from build123d import *

# Parameters (mm, degrees)
F0_R     = 7.5
F1_DEPTH = 10
F2_DEPTH = 30


with BuildPart() as f1:
    # F0 (on Front) → F1 (new body)
    with BuildSketch(Plane.XZ):
        with BuildLine():
            ThreePointArc((3, -19.77372), (15.165751, -13.038405), (20, 0))
            ThreePointArc((20, 0), (15.165751, 13.038405), (3, 19.77372))
            ThreePointArc((3, 19.77372), (-20, 0), (3, -19.77372))
        make_face()
        with BuildLine():
            Line((12.5, 3), (12.5, -3))
            Line((12.5, -3), (6.873864, -3))
            ThreePointArc((6.873864, -3), (0, -7.5), (-6.873864, -3))
            Line((-6.873864, -3), (-12.5, -3))
            Line((-12.5, -3), (-12.5, 3))
            Line((-12.5, 3), (-6.873864, 3))
            ThreePointArc((-6.873864, 3), (0, 7.5), (6.873864, 3))
            Line((6.873864, 3), (12.5, 3))
        make_face(mode=Mode.SUBTRACT)
        with BuildLine():
            ThreePointArc((3, 19.77372), (15.165751, 13.038405), (20, 0))
            ThreePointArc((20, 0), (15.165751, -13.038405), (3, -19.77372))
            Line((3, -19.77372), (51.875, -12.358575))
            ThreePointArc((51.875, -12.358575), (37.5, 0), (51.875, 12.358575))
            Line((51.875, 12.358575), (3, 19.77372))
        make_face()
        with BuildLine():
            ThreePointArc((62.5, 0), (59.478594, 8.149003), (51.875, 12.358575))
            ThreePointArc((51.875, 12.358575), (37.5, 0), (51.875, -12.358575))
            ThreePointArc((51.875, -12.358575), (59.478594, -8.149003), (62.5, 0))
        make_face()
        with Locations((50, 0)):
            Circle(F0_R, mode=Mode.SUBTRACT)
        with BuildLine():
            Line((-12.5, -3), (-6.873864, -3))
            ThreePointArc((-6.873864, -3), (-7.5, 0), (-6.873864, 3))
            Line((-6.873864, 3), (-12.5, 3))
            Line((-12.5, 3), (-12.5, -3))
        make_face()
    extrude(amount=F1_DEPTH)

    # F0 (on Front) → F2 (join)
    with BuildSketch(Plane.XZ):
        with BuildLine():
            ThreePointArc((3, -19.77372), (15.165751, -13.038405), (20, 0))
            ThreePointArc((20, 0), (15.165751, 13.038405), (3, 19.77372))
            ThreePointArc((3, 19.77372), (-20, 0), (3, -19.77372))
        make_face()
        with BuildLine():
            Line((12.5, 3), (12.5, -3))
            Line((12.5, -3), (6.873864, -3))
            ThreePointArc((6.873864, -3), (0, -7.5), (-6.873864, -3))
            Line((-6.873864, -3), (-12.5, -3))
            Line((-12.5, -3), (-12.5, 3))
            Line((-12.5, 3), (-6.873864, 3))
            ThreePointArc((-6.873864, 3), (0, 7.5), (6.873864, 3))
            Line((6.873864, 3), (12.5, 3))
        make_face(mode=Mode.SUBTRACT)
        with BuildLine():
            Line((-12.5, -3), (-6.873864, -3))
            ThreePointArc((-6.873864, -3), (-7.5, 0), (-6.873864, 3))
            Line((-6.873864, 3), (-12.5, 3))
            Line((-12.5, 3), (-12.5, -3))
        make_face()
    extrude(amount=F2_DEPTH)


solid = f1.part
Can you work these out from the model? Positions are in its coordinate system, mm. A direction names the side the tool comes from. Round coordinates to 2 decimals unless told otherwise and drop trailing zeros. Order: outer loops, then holes, each group sorted by start corner. A loop starts at its lowest first (then second) coordinate and runs counter-clockwise, first axis right, second up. Notation, with made-up numbers: (-7, 22) -> (38, 22) arc R24 cw to (38, 48) -> close; hole circle Ø6 at (24, 19.5). An arc over 180 degrees is marked (long way). Write each question's results on one line, items separated by ' | '. Start each with the question number.
Item 1: Thinking about a two-plate mould opening in Z: for faces 3 (the flat face through (27.095, -4.93, -16.118)), 4 (the flat face through (12.5, -15, 0)), 5 (the flat face through (32, -10, 0)), 6 (the flat face through (27.78, -4.93, 16.014)), which applies, +Z half, -Z half, draft (parallel to the pull), parting line (faces both ways), or undercut?
Item 2: If we section it at C-C, the plane z = 5.5: Write out the boundary of the cut face in (x, y).
Item 3: Please list where these lines run through material, in increasing order: L1, parallel to Y at x = 37.5, z = -0.5; L2, parallel to Z at x = 50, y = -2.25; L3, parallel to X at y = -16.5, z = 1.
Item 4: Which directions (+Z, -Z, +X, -X, +Y, -Y) give clear straight access to the entire face, cutting with the end or side of a thin tool? Please do faces 1 (the flat face through (21, 0, 0)), 2 (the flat face through (10, -15, -3)).
Item 5: If we section it at A-A, the plane x = -3: Write out the boundary of the cut face in (y, z).
Item 6: Will these pins go through, and if not, where does the flat tip stop? pin 1 (3 mm diameter, centred on x = 39.5, y = -3.5, fed in from +Z); pin 2 (5 mm diameter, centred on y = -6.5, z = 12, fed in from +X); pin 3 (3 mm diameter, centred on y = -13.5, z = 1, fed in from -X).
Item 7: If we section it at D-D, the plane y = -2.5: Write out the boundary of the cut face in (x, z) (3 decimals), then the cut area to 3 significant figures.
Item 8: If we section it at B-B, the plane y = -20: Write out the boundary of the cut face in (x, z), then the cut area to 3 significant figures.
Results:
1) face 3: -Z half | face 4: undercut | face 5: draft | face 6: +Z half
2) outline: (-19.23, -30) -> (-5.1, -30) -> (-5.1, 0) -> (-19.23, 0) -> close; (5.1, -30) -> (19.23, -30) -> (19.23, -10) -> (44.9, -10) -> (44.9, 0) -> (5.1, 0) -> close; (55.1, -10) -> (61.22, -10) -> (61.22, 0) -> (55.1, 0) -> close
3) L1: y = -10 to 0 | L2: z = -12.64 to -7.5, 7.5 to 12.64 | L3: x = -19.97 to -7.43, 12.5 to 19.97
4) face 1: +Z, -Z, +X, -X, +Y | face 2: +Y, -Y
5) outline: (-30, -19.77) -> (0, -19.77) -> (0, -6.87) -> (-30, -6.87) -> close; (-30, 6.87) -> (0, 6.87) -> (0, 19.77) -> (-30, 19.77) -> close
6) pin 1: stops at z = 14.46 | pin 2: stops at x = 58.12 | pin 3: stops at x = -20
7) outline: (3, -19.774) -> (51.875, -12.359) arc R12.5 ccw to (62.5, 0) arc R12.5 ccw to (51.875, 12.359) -> (3, 19.774) arc R20 ccw (long way) to start; hole (-6.874, -3) arc R7.5 ccw to (6.874, -3) -> (12.5, -3) -> (12.5, 3) -> (6.874, 3) arc R7.5 ccw to (-6.874, 3) arc R7.5 ccw to start; hole circle Ø15 at (50, 0) | area: 2,130 mm2
8) outline: (3, 19.77) arc R20 ccw (long way) to (20, 0) arc R20 ccw to start; hole (-6.87, -3) arc R7.5 ccw to (6.87, -3) -> (12.5, -3) -> (12.5, 3) -> (6.87, 3) arc R7.5 ccw to (-6.87, 3) arc R7.5 ccw to start | area: 1,050 mm2
